from build123d import *

# Parameters (mm, degrees)
F1_DEPTH = 3
F3_DEPTH = 3
F4_W     = 30
F4_H     = 6.25
F5_DEPTH = 6


with BuildPart() as f1:
    # F0 (on Right) → F1 (new body, symmetric)
    with BuildSketch(Plane.YZ):
        Polygon((23, -28), (23, 0), (-23, 0), (-23, -32.024479), align=None)
    extrude(amount=F1_DEPTH, both=True)

    # F2 (on Right) → F3 (join, symmetric)
    with BuildSketch(Plane.YZ):
        Polygon((-23, -32.024479), (-22.477066, -38.001647), (-11.929499, -37.078854), (-12.452434, -31.101686), align=None)
        Polygon((23.522934, -33.977168), (23, -28), (12.452434, -28.922792), (12.975368, -34.899961), align=None)
    extrude(amount=F3_DEPTH, both=True)

    # F4 (on face) → F5 (cut, through all)
    with BuildSketch(Plane.YZ.offset(3)):
        with Locations((0, -6.125)):
            Rectangle(F4_W, F4_H)
    extrude(amount=-F5_DEPTH, mode=Mode.SUBTRACT)


solid = f1.part
Work out the finished part from the listing and answer in its coordinate system (mm). A direction names the side the tool comes from. Give positions to 0.01 mm unless a question says otherwise; leave off trailing zeros. Order: outer loops, then holes, each group sorted by start corner. A loop starts at its lowest first (then second) coordinate and runs counter-clockwise, first axis right, second up. Notation, with made-up numbers: (13.25, 45) - (60.25, 45) arc R12 ccw to (60.25, 68) - close; hole circle Ø3 at (-22.75, 74.25). An arc over 180 degrees is marked (long way). Answer as CSV lines item,"result". Start each with the question number.
Q1. The part is cut by section C-C (y = -4.5). Write down the section's boundary in (x, z), then the cut area to 3 significant figures.
Q2. The mould has two halves that part along Z. Classify faces 4 (the face through (0, 23, -14)), 5 (the face through (0, 15, -6)), 6 (the face through (-0.042, -17.277, -37.547)): +Z half, -Z half, draft (parallel to the pull), parting line (faces both ways), or undercut.
Q3. Find the intervals of material crossed by L1, parallel to Y at x = 0.5, z = -6; L2, parallel to Y at x = 1.75, z = -21.5; L3, parallel to Z at x = 1.85, y = 6, in increasing order. Write a range as [from, to].
Q4. For faces 1 (the face through (0, -23, -16)), 2 (the face through (0, -15, -6)), 3 (the face through (0.04, 12.71, -31.87)), determine the directions among +Z, -Z, +X, -X, +Y, -Y from which every point of the face is accessible in a straight line to the end or side of a thin tool.
Q5. The part is cut by section B-B (x = -1.5). Write down the section's boundary in (y, z).
Q6. The part is cut by section A-A (z = -8). Write down the section's boundary in (x, y).
Q7. Given pin 1 Ø1.8 at (x, y) = (1.5, -0.5) entering from -Z; pin 2 Ø3 at (x, z) = (0.5, -10.5) entering from +Y; pin 3 Ø4 at (y, z) = (5.5, -6.5) entering from +X; pin 4 Ø1.8 at (x, y) = (0, 0.5) entering from +Z, each flat-ended and moving along its own axis, determine where each tip first touches the part or whether it passes through.
Check result:
1,outline,"(-3, -30.41) - (3, -30.41) - (3, -9.25) - (-3, -9.25) - close; (-3, -3) - (3, -3) - (3, 0) - (-3, 0) - close"
1,area,"145 mm²"
2,face 4,"draft"
2,face 5,"undercut"
2,face 6,"-Z half"
3,L1,"y = [-23, -15], [15, 23]"
3,L2,"y = [-23, 23]"
3,L3,"z = [-29.49, -9.25], [-3, 0]"
4,face 1,"+Z, -Z, +X, -X, -Y"
4,face 2,"+X, -X"
4,face 3,"-Z, +X, -X"
5,outline,"(-23, -32.02) - (-22.48, -38) - (-11.93, -37.08) - (-12.45, -31.1) - (12.45, -28.92) - (12.98, -34.9) - (23.52, -33.98) - (23, -28) - (23, 0) - (-23, 0) - close; hole (-15, -9.25) - (15, -9.25) - (15, -3) - (-15, -3) - close"
6,outline,"(-3, -23) - (3, -23) - (3, -15) - (-3, -15) - close; (-3, 15) - (3, 15) - (3, 23) - (-3, 23) - close"
7,pin 1,"stops at z = -30.13"
7,pin 2,"stops at y = 23"
7,pin 3,"passes through"
7,pin 4,"stops at z = 0"
